The model under review builds one solid part; all positions refer to its coordinate system, in mm. A direction names the side the tool comes from. Round coordinates to 2 decimals unless told otherwise and drop trailing zeros. Write each loop counter-clockwise with the first axis right and the second up, starting at its lowest first coordinate (ties: lowest second). Pieces come first, ordered by that corner, then holes. Notation, with made-up numbers: M 5,76.25 L 44,76.25 A18 cw 44,110.25 Z; hole C 86,-39 d8. An arc over 180 degrees is marked long. Write item = value, one per line. Start each with the question number.
Item 1: Take a section at C-C, the plane z = 9. Give the boundary of the cut face in (x, y), plus the area to 3 significant figures.
Item 2: Take a section at B-B, the plane x = 23.5. Give the boundary of the cut face in (y, z).
Item 3: Take a section at D-D, the plane x = 2. Give the boundary of the cut face in (y, z).
Item 4: For pin 1 Ø5 at (x, z) = (3, -2) entering from +Y; pin 2 Ø10 at (y, z) = (-12, 5.5) entering from +X; pin 3 Ø4 at (x, z) = (2.5, -2) entering from +Y, all flat-tipped, find the tip position at first contact; note any pin that passes through.
Item 5: To check wall thickness, follow line 1 along X through (y, z) = (-8.5, 11.5); line 2 along X through (y, z) = (0, 10); line 3 along Z through (x, y) = (21, -5.5). State the ranges of each line that lie inside material, in increasing order.
Item 6: Take a section at A-A, the plane z = 3. Give the boundary of the cut face in (x, y), plus the area to 3 significant figures.
Item 7: Tool access review of faces 1 (the flat face through (10, -6, 15)), 2 (the flat face through (0, -6, 15)), 3 (the cylindrical face through (18.98, -4.93, -2.73)): name each direction out of +Z, -Z, +X, -X, +Y, -Y from which nothing blocks a thin tool from reaching the whole face with its end or side.
from build123d import *

# Parameters (mm, degrees)
F0_R         = 3.75
F0_R_2       = 1.25
F1_DEPTH     = 10
F2_DEPTH     = 20
F3_DEPTH     = 30
F4_T1_DEPTH  = 23.936451485
F4_T3_DEPTH  = 23.936451485
F4_T8_DEPTH  = 23.936451485
F4_S9_R      = 1.25
F4_T10_DEPTH = 15
F4_T14_ANGLE = 156.4026846179
F4_S15_R     = 1.25
F4_T16_DEPTH = 8
F4_T18_ANGLE = 203.5973153821
F4_T22_DEPTH = 23.936451485
F4_S23_R     = 1.25
F4_T24_DEPTH = 15
F4_T26_ANGLE = 156.4026846179
F4_T28_ANGLE = 203.5973153821
F5_SIZE      = 1
F6_SIZE      = 0.5


# Not quite as in the source:
# - a fillet or chamfer that OpenCascade refuses, or shapes differently, is made with other operations: its cross-section is extruded or revolved along the edge and cut away or added


with BuildPart() as f1:
    # F0 (on Right) → F1 (new body)
    with BuildSketch(Plane.YZ):
        with BuildLine():
            ThreePointArc((3.6919470815, 19.2276737533), (3.8502654993, 20.2445960951), (3.9032252878, 21.2724049449))
            ThreePointArc((3.9032252878, 21.2724049449), (-7.124583562, 31.2194451563), (-15.8854965059, 19.2276737533))
            ThreePointArc((-15.8854965059, 19.2276737533), (-6.0967747122, 11.2724049449), (3.6919470815, 19.2276737533))
        make_face()
        with Locations((-6.0967747122, 21.2724049449)):
            Circle(F0_R, mode=Mode.SUBTRACT)
        with BuildLine():
            ThreePointArc((3.6919470815, 19.2276737533), (-6.0967747122, 11.2724049449), (-15.8854965059, 19.2276737533))
            Line((-15.8854965059, 19.2276737533), (-10.991135609, -4.2030526781))
            ThreePointArc((-10.991135609, -4.2030526781), (-6.6106791371, 1.7928330234), (-1.0967747122, -3.1806870823))
            ThreePointArc((-1.0967747122, -3.1806870823), (-1.1232546065, -3.6945915072), (-1.2024138154, -4.2030526781))
            Line((-1.2024138154, -4.2030526781), (3.6919470815, 19.2276737533))
        make_face()
        with BuildLine():
            ThreePointArc((-1.0967747122, -3.1806870823), (-6.6106791371, 1.7928330234), (-10.991135609, -4.2030526781))
            ThreePointArc((-10.991135609, -4.2030526781), (-6.0967747122, -8.1806870823), (-1.2024138154, -4.2030526781))
            ThreePointArc((-1.2024138154, -4.2030526781), (-1.1232546065, -3.6945915072), (-1.0967747122, -3.1806870823))
        make_face()
        with Locations((-6.0967747122, -3.1806870823)):
            Circle(F0_R_2, mode=Mode.SUBTRACT)
        with Locations((-6.0967747122, 21.2724049449)):
            Circle(F0_R)
        with Locations((-6.0967747122, -3.1806870823)):
            Circle(F0_R_2)
    extrude(amount=F1_DEPTH)

    # F0 (on Right) → F2 (join)
    with BuildSketch(Plane.YZ):
        with Locations((-6.0967747122, 21.2724049449)):
            Circle(F0_R)
    extrude(amount=-F2_DEPTH)

    # F0 (on Right) → F3 (join)
    with BuildSketch(Plane.YZ):
        with Locations((-6.0967747122, -3.1806870823)):
            Circle(F0_R_2)
    extrude(amount=F3_DEPTH)

    # F4: chamfer of 5 on 2 edges, made by hand

    # F4_s2 → F4_t1 (cut)
    with BuildSketch(Plane(origin=(0, -0.8915258311, -4.2679929606), x_dir=(1, 0, 0), z_dir=(0, 0.2044731192, 0.9788721794))):
        Polygon((5, -0.3175981408), (0, -5.3175981408), (0, -0.3175981408), align=None)
    extrude(amount=F4_T1_DEPTH, mode=Mode.SUBTRACT)

    # F4_s4 → F4_t3 (cut)
    with BuildSketch(Plane(origin=(0, -4.5126383008, 21.6033095513), x_dir=(1, 0, 0), z_dir=(0, 0.2044731192, -0.9788721794))):
        Polygon((5, 11.6183281585), (0, 6.6183281585), (0, 11.6183281585), align=None)
    extrude(amount=F4_T3_DEPTH, mode=Mode.SUBTRACT)


with BuildPart() as f4_tool6:
    # F4_s7 → F4_t8 (new body)
    with BuildSketch(Plane(origin=(0, -0.8915258311, -4.2679929606), x_dir=(1, 0, 0), z_dir=(0, 0.2044731192, 0.9788721794))):
        Polygon((5, -0.3175981408), (10, -5.3175981408), (10, -0.3175981408), align=None)
    extrude(amount=F4_T8_DEPTH)

    # F4_s9 → F4_t10 (cut, symmetric)
    with BuildSketch(Plane.YZ.offset(7.5)):
        with Locations((-6.0967747122, -3.1806870823)):
            Circle(F4_S9_R)
    extrude(amount=F4_T10_DEPTH, both=True, mode=Mode.SUBTRACT)


with BuildPart() as f1_1:
    add(f1.part)

    # F4_t5: cut F4_tool6
    add(f4_tool6.part, mode=Mode.SUBTRACT)


with BuildPart() as f4_tool12:
    # F4_s13 → F4_t14 (revolve)
    with BuildSketch(Plane(origin=(0, 0.381722596, -1.8274168801), x_dir=(1, 0, 0), z_dir=(0, -0.2044731192, 0.9788721794))):
        Polygon((10, -6.6183281585), (5, -11.6183281585), (10, -11.6183281585), align=None)
    revolve(axis=Axis((10, -6.0967747122, -3.1806870823), (1, 0, 0)), revolution_arc=F4_T14_ANGLE)

    # F4_s15 → F4_t16 (cut, symmetric)
    with BuildSketch(Plane.YZ.offset(7.5)):
        with Locations((-6.0967747122, -3.1806870823)):
            Circle(F4_S15_R)
    extrude(amount=F4_T16_DEPTH, both=True, mode=Mode.SUBTRACT)


with BuildPart() as f1_2:
    add(f1_1.part)

    # F4_t11: cut F4_tool12
    add(f4_tool12.part, mode=Mode.SUBTRACT)

    # F4_s17 → F4_t18 (revolve, cut)
    with BuildSketch(Plane(origin=(0, 4.0028350658, 19.1627334708), x_dir=(1, 0, 0), z_dir=(0, -0.2044731192, -0.9788721794))):
        Polygon((5, 0.3175981408), (10, 5.3175981408), (10, 0.3175981408), align=None)
    revolve(axis=Axis((10, -6.0967747122, 21.2724049449), (1, 0, 0)), revolution_arc=F4_T18_ANGLE, mode=Mode.SUBTRACT)


with BuildPart() as f4_tool20:
    # F4_s21 → F4_t22 (new body)
    with BuildSketch(Plane(origin=(0, -4.5126383008, 21.6033095513), x_dir=(1, 0, 0), z_dir=(0, 0.2044731192, -0.9788721794))):
        Polygon((5, 11.6183281585), (10, 6.6183281585), (10, 11.6183281585), align=None)
    extrude(amount=F4_T22_DEPTH)

    # F4_s23 → F4_t24 (cut, symmetric)
    with BuildSketch(Plane.YZ.offset(7.5)):
        with Locations((-6.0967747122, -3.1806870823)):
            Circle(F4_S23_R)
    extrude(amount=F4_T24_DEPTH, both=True, mode=Mode.SUBTRACT)


with BuildPart() as f1_3:
    add(f1_2.part)

    # F4_t19: cut F4_tool20
    add(f4_tool20.part, mode=Mode.SUBTRACT)

    # F4_s25 → F4_t26 (revolve, cut)
    with BuildSketch(Plane(origin=(0, 0.381722596, -1.8274168801), x_dir=(1, 0, 0), z_dir=(0, -0.2044731192, 0.9788721794))):
        Polygon((0, -6.6183281585), (5, -11.6183281585), (0, -11.6183281585), align=None)
    revolve(axis=Axis((0, -6.0967747122, -3.1806870823), (1, 0, 0)), revolution_arc=F4_T26_ANGLE, mode=Mode.SUBTRACT)

    # F4_s27 → F4_t28 (revolve, cut)
    with BuildSketch(Plane(origin=(0, 4.0028350658, 19.1627334708), x_dir=(1, 0, 0), z_dir=(0, -0.2044731192, -0.9788721794))):
        Polygon((5, 0.3175981408), (0, 5.3175981408), (0, 0.3175981408), align=None)
    revolve(axis=Axis((0, -6.0967747122, 21.2724049449), (1, 0, 0)), revolution_arc=F4_T28_ANGLE, mode=Mode.SUBTRACT)

    # F5
    f5_edges = [f1_3.edges().sort_by_distance(p)[0] for p in [
        (-20, -9.846775, 21.272405),
    ]]
    chamfer(f5_edges, length=F5_SIZE)

    # F6
    f6_edges = [f1_3.edges().sort_by_distance(p)[0] for p in [
        (30, -7.346775, -3.180687),
    ]]
    chamfer(f6_edges, length=F6_SIZE)


solid = f1_3.part
Response values:
q1.outline = M 0,-8.64 L 5,-13.75 L 10,-8.64 L 10,-3.55 L 5,1.56 L 0,-3.55 Z
q1.area = 102 mm2
q2.outline = C -6.1,-3.18 d2.5
q3.outline = M -12.95,19.84 L -8.05,-3.59 A2 ccw -4.14,-3.59 L 0.76,19.84 A7 ccw long Z
q4.pin_1 = -0.43
q4.pin_2 = 10
q4.pin_3 = -1.21
q5.line_1 = 0 to 10
q5.line_2 = 3.27 to 6.73
q5.line_3 = -4.28 to -2.08
q6.outline = M 0,-7.39 L 5,-12.5 L 10,-7.39 L 10,-4.81 L 5,0.3 L 0,-4.81 Z
q6.area = 76.9 mm2
q7.face_1 = +Z, +X, +Y, -Y
q7.face_2 = -X
q7.face_3 = +X
